Geometry: final body of the model. Coordinates: model frame, mm. Round coordinates to 2 decimals unless told otherwise and drop trailing zeros. Write each loop counter-clockwise with the first axis right and the second up, starting at its lowest first coordinate (ties: lowest second). Pieces come first, ordered by that corner, then holes. Notation, with made-up numbers: M 2.5,-28 L 29.5,-28 A21 cw 29.5,8 Z; hole C 26.25,-14 d6. An arc over 180 degrees is marked long. Use one line per item in the form item = value. Start each with the question number.
Item 1: Section query A-A (z = 58). Return loops of the section in (x, y) (1 decimal).
Item 2: Pin query (flat end, axial travel): pin 1 Ø7.5 at (x, y) = (0, 0) entering from -Z; pin 2 Ø3 at (x, z) = (-3.5, 12.5) entering from +Y; pin 3 Ø4 at (x, y) = (-0.5, 1.5) entering from -Z. Return the tip coordinate at first contact, or that it passes through.
Item 3: Ray query, probe 1 along Y at (x, z) = (0, 119.5); probe 2 along Y at (x, z) = (3.75, 114); probe 3 along X at (y, z) = (0.25, 23). Return the intervals inside material, ascending.
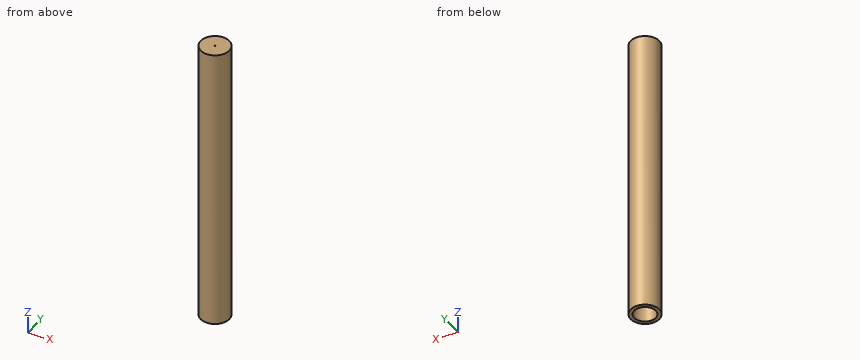
from build123d import *

# Parameters (mm, degrees)
F0_R     = 6.3603951
F1_DEPTH = 127
F2_D     = 9.525
F2_DEPTH = 114.3
F2_TIP   = 2.8615986981
F3_D     = 0.3302


with BuildPart() as f1:
    # F0 (on Top) → F1 (new body)
    with BuildSketch(Plane.XY):
        Circle(F0_R)
    extrude(amount=F1_DEPTH)

    # F2
    with Locations(Plane(origin=(0, 0, 0), x_dir=(1, 0, 0), z_dir=(0, 0, -1))):
        with Locations((0, 0)):
            Hole(F2_D / 2, depth=F2_DEPTH)
            with Locations((0, 0, -(F2_DEPTH + F2_TIP / 2))):  # 118° drill point
                Cone(0, F2_D / 2, F2_TIP, mode=Mode.SUBTRACT)

    # F3 (through all)
    with Locations(Plane(origin=(0, 0, 0), x_dir=(1, 0, 0), z_dir=(0, 0, -1))):
        with Locations((0, 0)):
            Hole(F3_D / 2)


solid = f1.part
Working result:
q1.outline = C 0,0 d12.7; hole C 0,0 d9.5
q2.pin_1 = 114.91
q2.pin_2 = 6.04
q2.pin_3 = 115.01
q3.probe_1 = -6.36 to -0.17, 0.17 to 6.36
q3.probe_2 = -5.14 to -2.94, 2.94 to 5.14
q3.probe_3 = -6.36 to -4.76, 4.76 to 6.36
